Here's how the part is built. I have some questions about the finished solid (model axes, mm). Round coordinates to 2 decimals unless told otherwise and drop trailing zeros. Write each loop counter-clockwise with the first axis right and the second up, starting at its lowest first coordinate (ties: lowest second). Pieces come first, ordered by that corner, then holes. Notation, with made-up numbers: (13.5, -13.75) -> (26.5, -13.75) arc R20 cw to (26.5, 8.25) -> close; hole circle Ø1 at (86.5, 38.5). An arc over 180 degrees is marked (long way). Put each result on its own line as item: value. Start each with the question number.
1. Suppose I cut it at D-D (z = -613.5). Please give me the cut outline in (x, y), then the cut area to 3 significant figures.
2. For pin 1 (14 mm diameter, centred on x = 2053.5, y = 400, fed in from -Z); pin 2 (5 mm diameter, centred on y = 840, z = -64, fed in from +X), each with a flat end and sliding along its axis, tell me the tip position at first contact or that it passes through.
3. Suppose I cut it at C-C (z = -239.5). Please give me the cut outline in (x, y), then the cut area to 3 significant figures.
4. Suppose I cut it at A-A (y = 271). Please give me the cut outline in (x, z), then the cut area to 3 significant figures.
5. I need wall thicknesses on probe 1 along Y at (x, z) = (301.5, -466.5); probe 2 along X at (y, z) = (542, -32); probe 3 along X at (y, z) = (721, -78). Which ranges of each line are inside material? Lowest first, please. Write a range as from..to.
6. Suppose I cut it at B-B (x = 474). Please give me the cut outline in (y, z), then the cut area to 3 significant figures.
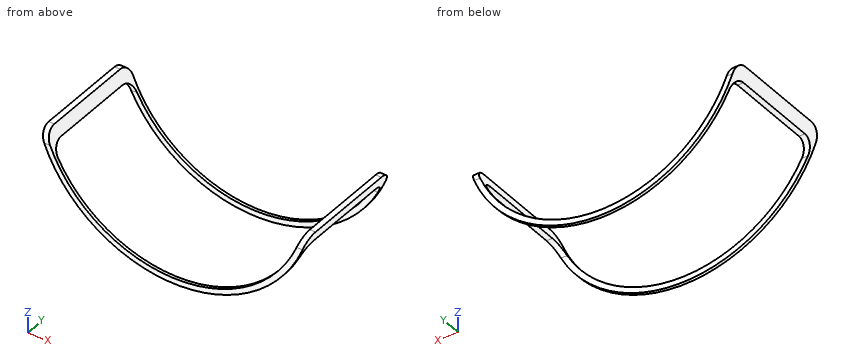
```python
from build123d import *

# Parameters (mm, degrees)
BOSS_EXTRUDE2_DEPTH = 950
FILLET2_R           = 100
CUT_EXTRUDE3_DEPTH  = 900
FILLET3_R           = 100


with BuildPart() as part:
    # Sketch2 → Boss-Extrude2 (new body)
    with BuildSketch(Plane(origin=(0, 0, 0), x_dir=(1, 0, 0), z_dir=(0, 1, 0))):
        with BuildLine():
            Line((2122.868885508, -17), (2076.979866157, -17))
            ThreePointArc((2076.979866157, -17), (1050, 745.128073785), (23.020133843, -17))
            Line((23.020133843, -17), (-22.868885508, -17))
            ThreePointArc((-22.868885508, -17), (1050, 789.128073785), (2122.868885508, -17))
        make_face()
    extrude(amount=BOSS_EXTRUDE2_DEPTH)

    # Fillet2
    fillet2_edges = [part.edges().sort_by_distance(p)[0] for p in [
        (2099.924375832, 950, 17),
        (0.075624168, 950, 17),
        (2099.924375832, 0, 17),
        (0.075624168, 0, 17),
    ]]
    fillet(fillet2_edges, radius=FILLET2_R)

    # Sketch4 → Cut-Extrude3 (cut)
    with BuildSketch(Plane(origin=(0, 25, 0), x_dir=(-1, 0, 0), z_dir=(0, -1, 0))):
        with BuildLine():
            Line((-2088.688240161, 83), (-2041.218068968, 83))
            ThreePointArc((-2041.218068968, 83), (-1050, 745.128073785), (-58.781931032, 83))
            Line((-58.781931032, 83), (-11.311759839, 83))
            ThreePointArc((-11.311759839, 83), (-1050, 789.128073785), (-2088.688240161, 83))
        make_face()
    extrude(amount=-CUT_EXTRUDE3_DEPTH, mode=Mode.SUBTRACT)

    # Fillet3
    fillet3_edges = [part.edges().sort_by_distance(p)[0] for p in [
        (35.046845436, 925, -83),
        (2064.953154564, 925, -83),
        (2064.953154564, 25, -83),
        (35.046845436, 25, -83),
    ]]
    fillet(fillet3_edges, radius=FILLET3_R)


solid = part.part
```
Verdict:
1. outline: (448.74, 0) -> (535.07, 0) -> (535.07, 25) -> (448.74, 25) -> close; (448.74, 925) -> (535.07, 925) -> (535.07, 950) -> (448.74, 950) -> close; (1564.93, 0) -> (1651.26, 0) -> (1651.26, 25) -> (1564.93, 25) -> close; (1564.93, 925) -> (1651.26, 925) -> (1651.26, 950) -> (1564.93, 950) -> close
1. area: 8,630 mm^2
2. pin 1: stops at z = -83
2. pin 2: stops at x = 2096.94
3. outline: (87.83, 0) -> (139.28, 0) -> (139.28, 25) -> (87.83, 25) -> close; (87.83, 925) -> (139.28, 925) -> (139.28, 950) -> (87.83, 950) -> close; (1960.72, 0) -> (2012.17, 0) -> (2012.17, 25) -> (1960.72, 25) -> close; (1960.72, 925) -> (2012.17, 925) -> (2012.17, 950) -> (1960.72, 950) -> close
3. area: 5,140 mm^2
4. outline: (-22.87, 17) arc R1117 ccw to (11.31, -83) -> (58.78, -83) arc R1073 cw to (23.02, 17) -> close; (2041.22, -83) -> (2088.69, -83) arc R1117 ccw to (2122.87, 17) -> (2076.98, 17) arc R1073 cw to start
4. area: 9,330 mm^2
5. probe 1: y = 0..25, 925..950
5. probe 2: x = -7.44..39.15, 2060.85..2107.44
5. probe 3: x = 9.35..56.72, 2043.28..2090.65
6. outline: (0, -629.16) -> (25, -629.16) -> (25, -577.42) -> (0, -577.42) -> close; (925, -629.16) -> (950, -629.16) -> (950, -577.42) -> (925, -577.42) -> close
6. area: 2,590 mm^2
